```python
from build123d import *

# Parameters (mm, degrees)
SKETCH_1_R      = 10.101525446
SKETCH_1_R_2    = 1.565736444
EXTRUDE_1_DEPTH = 2.5
SKETCH_2_R      = 4.5
SKETCH_2_R_2    = 3
EXTRUDE_2_DEPTH = 2


with BuildPart() as part:
    # 草图1 → 凸台-拉伸1 (new body)
    with BuildSketch(Plane.XY):
        Circle(SKETCH_1_R)
        Circle(SKETCH_1_R_2, mode=Mode.SUBTRACT)
        with Locations((7.071067812, 0)):
            Circle(SKETCH_1_R_2, mode=Mode.SUBTRACT)
        with Locations((-7.071067812, 0)):
            Circle(SKETCH_1_R_2, mode=Mode.SUBTRACT)
        with Locations((0, 7.071067812)):
            Circle(SKETCH_1_R_2, mode=Mode.SUBTRACT)
        with Locations((0, -7.071067812)):
            Circle(SKETCH_1_R_2, mode=Mode.SUBTRACT)
    extrude(amount=EXTRUDE_1_DEPTH)

    # 草图2 → 凸台-拉伸2 (add)
    with BuildSketch(Plane(origin=(0, 0, 0), x_dir=(-1, 0, 0), z_dir=(0, 0, -1))):
        Circle(SKETCH_2_R)
        Circle(SKETCH_2_R_2, mode=Mode.SUBTRACT)
    extrude(amount=EXTRUDE_2_DEPTH)


solid = part.part
```
Verification items for the finished model (mm, model axes). A direction names the side the tool comes from. Round coordinates to 2 decimals unless told otherwise and drop trailing zeros. Loops run counter-clockwise (first coordinate to the right, second up) from the corner with the lowest first, then second, coordinate; pieces in that order, holes last. Notation, with made-up numbers: (1.25, 85.5) -> (34.25, 85.5) arc R11 ccw to (34.25, 103.5) -> close; hole circle Ø9 at (14, 78.25). An arc over 180 degrees is marked (long way). Answer as a JSON object with one key per item and string values.
Q1. Section check A-A (x = 0). Record the boundary of the cut face in (y, z), then the cut area to 3 significant figures.
Data:
{"outline": "(-10.1, 0) -> (-8.64, 0) -> (-8.64, 2.5) -> (-10.1, 2.5) -> close; (-5.51, 0) -> (-4.5, 0) -> (-4.5, -2) -> (-3, -2) -> (-3, 0) -> (-1.57, 0) -> (-1.57, 2.5) -> (-5.51, 2.5) -> close; (1.57, 0) -> (3, 0) -> (3, -2) -> (4.5, -2) -> (4.5, 0) -> (5.51, 0) -> (5.51, 2.5) -> (1.57, 2.5) -> close; (8.64, 0) -> (10.1, 0) -> (10.1, 2.5) -> (8.64, 2.5) -> close", "area": "33.0 mm2"}
Q2. Draft check along X on faces 1 (the flat face through (0, -2, 2.5)), 2 (the cylindrical face through (-7.445, 6.827, 1.232)), 3 (the cylindrical face through (0.84, -5.75, 1.23)). Enter one of: pulls with the +X half, pulls with the -X half, needs draft (parallel to the pull), parting line crosses it, or undercut.
Data:
{"face 1": "needs draft", "face 2": "parting line crosses it", "face 3": "undercut"}
Q3. Go/stop test with flat-tipped pins: P1, Ø1.8, axis at x = 0.5, y = -1.5, coming from the -Z side; P2, Ø1.9, axis at x = -7.07, y = 0, coming from the -Z side. Record where each tip stops, or that it passes through.
Data:
{"P1": "stops at z = 0", "P2": "passes through"}
Q4. Scan lines: line 1 (Y direction, x = 0, z = 1.7); line 2 (Z direction, x = -3.25, y = 8); line 3 (Y direction, x = 0, z = -1.45). Record each from-to range of solid material in increasing order. Write a range as from..to.
Data:
{"line 1": "y = -10.1..-8.64, -5.51..-1.57, 1.57..5.51, 8.64..10.1", "line 2": "z = 0..2.5", "line 3": "y = -4.5..-3, 3..4.5"}
Q5. Section check C-C (x = -6.5). Record the boundary of the cut face in (y, z).
Data:
{"outline": "(-7.73, 0) -> (-1.46, 0) -> (-1.46, 2.5) -> (-7.73, 2.5) -> close; (1.46, 0) -> (7.73, 0) -> (7.73, 2.5) -> (1.46, 2.5) -> close"}
Q6. Section check D-D (y = -7.5). Record the boundary of the cut face in (x, z), then the cut area to 3 significant figures.
Data:
{"outline": "(-6.77, 0) -> (-1.51, 0) -> (-1.51, 2.5) -> (-6.77, 2.5) -> close; (1.51, 0) -> (6.77, 0) -> (6.77, 2.5) -> (1.51, 2.5) -> close", "area": "26.3 mm2"}
Q7. Access from +Z, -Z, +X, -X, +Y, -Y to the whole of each face (thin tool, end or side, straight path). Record for faces 4 (the cylindrical face through (0.59, 4.46, -0.99)), 5 (the flat face through (-1, -3, -2)).
Data:
{"face 4": "-Z", "face 5": "-Z, +X, -X, +Y, -Y"}
